Geometry check sheet. Reference: the model listing, model coordinates, mm. A direction names the side the tool comes from. Round coordinates to 2 decimals unless told otherwise and drop trailing zeros. Write each loop counter-clockwise with the first axis right and the second up, starting at its lowest first coordinate (ties: lowest second). Pieces come first, ordered by that corner, then holes. Notation, with made-up numbers: (66.25, 12) - (110.25, 12) arc R36 cw to (110.25, 50) - close; hole circle Ø9 at (17.5, 36.5). An arc over 180 degrees is marked (long way). Return JSON: item names as keys, results as strings.
```python
from build123d import *

# Parameters (mm, degrees)
SCHIZZO1_W                   = 121
SCHIZZO1_H                   = 56
ESTRUSIONE_ESTRUSIONE4_DEPTH = 51
SCHIZZO6_W                   = 118
SCHIZZO6_H                   = 48
TAGLIO_ESTRUSIONE2_DEPTH     = 53
SCHIZZO7_W                   = 22
SCHIZZO7_H                   = 28
ESTRUSIONE_ESTRUSIONE5_DEPTH = 48
SCHIZZO13_W                  = 20
SCHIZZO13_H                  = 26
TAGLIO_ESTRUSIONE3_DEPTH     = 48
SCHIZZO15_W                  = 118
SCHIZZO15_H                  = 1
ESTRUSIONE_ESTRUSIONE6_DEPTH = 2
SCHIZZO16_W                  = 3
SCHIZZO16_H                  = 1
ESTRUSIONE_ESTRUSIONE7_DEPTH = 48
SCHIZZO17_W                  = 49.5
SCHIZZO17_H                  = 1.75
TAGLIO_ESTRUSIONE4_DEPTH     = 120


with BuildPart() as part:
    # Schizzo1 → Estrusione-Estrusione4 (new body)
    with BuildSketch(Plane.XY):
        with Locations((60.5, 28)):
            Rectangle(SCHIZZO1_W, SCHIZZO1_H)
    extrude(amount=ESTRUSIONE_ESTRUSIONE4_DEPTH)

    # Schizzo6 → Taglio-Estrusione2 (cut)
    with BuildSketch(Plane.XZ):
        with Locations((60.5, 25.5)):
            Rectangle(SCHIZZO6_W, SCHIZZO6_H)
    extrude(amount=-TAGLIO_ESTRUSIONE2_DEPTH, mode=Mode.SUBTRACT)

    # Schizzo7 → Estrusione-Estrusione5 (add)
    with BuildSketch(Plane.XZ.offset(-53)):
        with Locations((12.5, 35.5)):
            Rectangle(SCHIZZO7_W, SCHIZZO7_H)
    extrude(amount=ESTRUSIONE_ESTRUSIONE5_DEPTH)

    # Schizzo13 → Taglio-Estrusione3 (cut)
    with BuildSketch(Plane.XZ.offset(-5)):
        with Locations((12.5, 35.5)):
            Rectangle(SCHIZZO13_W, SCHIZZO13_H)
    extrude(amount=-TAGLIO_ESTRUSIONE3_DEPTH, mode=Mode.SUBTRACT)

    # Schizzo15 → Estrusione-Estrusione6 (add)
    with BuildSketch(Plane.XZ.offset(-53)):
        with Locations((60.5, 7)):
            Rectangle(SCHIZZO15_W, SCHIZZO15_H)
    extrude(amount=ESTRUSIONE_ESTRUSIONE6_DEPTH)

    # Schizzo16 → Estrusione-Estrusione7 (add)
    with BuildSketch(Plane.XZ.offset(-51)):
        with Locations((118, 7)):
            Rectangle(SCHIZZO16_W, SCHIZZO16_H)
    extrude(amount=ESTRUSIONE_ESTRUSIONE7_DEPTH)

    # Schizzo17 → Taglio-Estrusione4 (cut)
    with BuildSketch(Plane(origin=(121, 0, 0), x_dir=(0, 0, -1), z_dir=(1, 0, 0))):
        with Locations((-25.5, 1.875)):
            Rectangle(SCHIZZO17_W, SCHIZZO17_H)
    extrude(amount=-TAGLIO_ESTRUSIONE4_DEPTH, mode=Mode.SUBTRACT)


solid = part.part
```
(1) Section check A-A, the plane y = 8. Enter the section's corners in (x, z), plus the area to 3 significant figures.
Response values:
{"outline": "(0, 0) - (121, 0) - (121, 51) - (0, 51) - close; hole (1.5, 1.5) - (119.5, 1.5) - (119.5, 6.5) - (116.5, 6.5) - (116.5, 7.5) - (119.5, 7.5) - (119.5, 49.5) - (23.5, 49.5) - (23.5, 21.5) - (1.5, 21.5) - close; hole (2.5, 22.5) - (22.5, 22.5) - (22.5, 48.5) - (2.5, 48.5) - close", "area": "606 mm^2"}
(2) Access from +Z, -Z, +X, -X, +Y, -Y to the whole of each face (thin tool, end or side, straight path). Record for faces 4 (the face through (60, 0, 1)), 5 (the face through (1.5, 28, 9)).
Response values:
{"face 4": "+Z, -Z, +X, -X, -Y", "face 5": "-Y"}
(3) Section check D-D, the plane z = 26. Enter the section's corners in (x, y), plus the area to 4 significant figures.
Response values:
{"outline": "(0, 0) - (1.5, 0) - (1.5, 1) - (1, 1) - (1, 2.75) - (1.5, 2.75) - (1.5, 5) - (2.5, 5) - (2.5, 53) - (22.5, 53) - (22.5, 5) - (23.5, 5) - (23.5, 53) - (119.5, 53) - (119.5, 2.75) - (121, 2.75) - (121, 56) - (0, 56) - close; (119.5, 0) - (121, 0) - (121, 1) - (119.5, 1) - close", "area": "614.5 mm^2"}
(4) Section check B-B, the plane z = 17.5. Enter the section's corners in (x, y).
Response values:
{"outline": "(0, 0) - (1.5, 0) - (1.5, 1) - (1, 1) - (1, 2.75) - (1.5, 2.75) - (1.5, 53) - (119.5, 53) - (119.5, 2.75) - (121, 2.75) - (121, 56) - (0, 56) - close; (119.5, 0) - (121, 0) - (121, 1) - (119.5, 1) - close"}
(5) Section check C-C, the plane x = 58. Enter the section's corners in (y, z), plus the area to 3 significant figures.
Response values:
{"outline": "(0, 0) - (56, 0) - (56, 51) - (0, 51) - (0, 49.5) - (1, 49.5) - (1, 50.25) - (2.75, 50.25) - (2.75, 49.5) - (53, 49.5) - (53, 7.5) - (51, 7.5) - (51, 6.5) - (53, 6.5) - (53, 1.5) - (2.75, 1.5) - (2.75, 0.75) - (1, 0.75) - (1, 1.5) - (0, 1.5) - close", "area": "311 mm^2"}
(6) Release check for a two-part mould opening along Z. For faces 1 (the face through (60, 28, 51)), 2 (the face through (119.5, 28, 25)), 3 (the face through (60, 56, 25)) record: pulls with the +Z half, pulls with the -Z half, needs draft (parallel to the pull), parting line crosses it, or undercut.
Response values:
{"face 1": "pulls with the +Z half", "face 2": "undercut", "face 3": "needs draft"}
(7) Material ranges on line 1 along X through (y, z) = (43.5, 32); line 2 along Z through (x, y) = (23, 52.5); line 3 along Z through (x, y) = (36.5, 49.5), recorded low to high. Write a range as [from, to].
Response values:
{"line 1": "x = [0, 2.5], [22.5, 23.5], [119.5, 121]", "line 2": "z = [0, 1.5], [6.5, 7.5], [21.5, 51]", "line 3": "z = [0, 1.5], [49.5, 51]"}
(8) Gauge pin test, flat ends, axial feed: pin 1 (1.5 mm diameter, centred on x = 36, y = 21.5, fed in from -Z); pin 2 (25 mm diameter, centred on x = 58.5, z = 16, fed in from -Y); pin 3 (1.4 mm diameter, centred on y = 2, z = 27.5, fed in from +X); pin 4 (2.5 mm diameter, centred on x = 72.5, z = 3, fed in from -Y). Record the tip position at first contact, or that the pin passes through.
Response values:
{"pin 1": "stops at z = 0", "pin 2": "stops at y = 51", "pin 3": "stops at x = 1", "pin 4": "stops at y = 53"}
